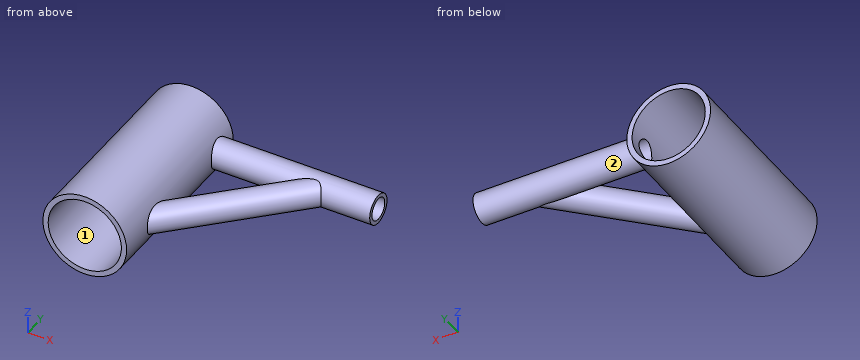
from build123d import *

# Parameters (mm, degrees)
F0_R          = 29.0718319872
F1_DEPTH      = 63.5
F3_D          = 50.8
F6_R          = 10.3012460199
F7_DEPTH      = 110.01212
F7_DEPTH_BACK = 2.28984
F11_START     = 10.10954
F10_R         = 9.3240211729
F11_DEPTH     = 116.89046
F13_D         = 15.24
F13_DEPTH     = 127
F13_TIP       = 4.578557917
F14_R         = 25.4
F15_DEPTH     = 127


with BuildPart() as f1:
    # F0 (on Front) → F1 (new body, symmetric)
    with BuildSketch(Plane.XZ):
        Circle(F0_R)
    extrude(amount=F1_DEPTH, both=True)

    # F3 (through all)
    with Locations(Plane.XZ.offset(63.5)):
        with Locations((0, 0)):
            Hole(F3_D / 2)

    # F6 (on plane+point) → F7 (join, two sides)
    with BuildSketch(Plane.YZ.offset(29.0718319872)) as f7_sk:
        with Locations((47.6702228189, 0)):
            Circle(F6_R)
    extrude(amount=F7_DEPTH)
    extrude(f7_sk.sketch, amount=-F7_DEPTH_BACK)

    # F10 (on line) → F11 (join)
    with BuildSketch(Plane(origin=(-16.7531975657, -16.7531975657, 0), x_dir=(-0.7071067812, 0.7071067812, 0), z_dir=(0.7071067812, 0.7071067812, 0)).offset(F11_START)):
        with Locations((-38.7535318732, 0)):
            Circle(F10_R)
    extrude(amount=F11_DEPTH)

    # F13
    with Locations(Plane.YZ.offset(139.0839519872)):
        with Locations((47.6702228189, 0)):
            Hole(F13_D / 2, depth=F13_DEPTH)
            with Locations((0, 0, -(F13_DEPTH + F13_TIP / 2))):  # 118° drill point
                Cone(0, F13_D / 2, F13_TIP, mode=Mode.SUBTRACT)

    # F14 (on Front) → F15 (cut)
    with BuildSketch(Plane.XZ):
        Circle(F14_R)
    extrude(amount=F15_DEPTH, mode=Mode.SUBTRACT)


solid = f1.part
Design review of the part built by this model. Coordinates are the model's own, in mm. Face numbers are marked on the shaded views. A direction names the side the tool comes from. Coordinates: 2 decimals unless noted, no trailing zeros. Loops run counter-clockwise (first coordinate to the right, second up) from the corner with the lowest first, then second, coordinate; pieces in that order, holes last. Notation, with made-up numbers: (8.25, 34.5) -> (64.25, 34.5) arc R11 ccw to (64.25, 38.5) -> close; hole circle Ø7 at (69.25, 1). An arc over 180 degrees is marked (long way). Use a Markdown table: item, result. Add a question column.
Item 1: We need section A-A, the plane z = -2.5. Write out the cut boundary in (x, y), and give its area (3 significant figures).
Item 2: We need section B-B, the plane x = 0. Write out the cut boundary in (y, z).
Item 3: We need section D-D, the plane y = -52. Write out the cut boundary in (x, z).
Item 4: We need section C-C, the plane z = 22. Write out the cut boundary in (x, y).
Item 5: Clearance check with flat-ended pins moving along their axes: P1, Ø12, axis at y = -30, z = -11.5, coming from the +X side; P2, Ø3, axis at x = 73, z = 4, coming from the +Y side; P3, Ø2, axis at x = 64, z = -6, coming from the -Y side. State where each tip first meets the part, or that it passes through.
Item 6: Wall thickness on L1, parallel to Y at x = 34.5, z = -3; L2, parallel to Z at x = 0, y = 3; L3, parallel to Y at x = 114, z = 0: over which ranges is each line inside the solid? List them lowest first. Write a range as from..to.
Item 7: Machinability: for the marked faces 1 and 2, which of the approach directions +Z, -Z, +X, -X, +Y, -Y give a long, thin tool a straight path to every point of the face, cutting with its end or side? Answer none if there is none.
Numbers:
| question | item | result |
|---|---|---|
| 1 | outline | (-28.96, -63.5) -> (-25.28, -63.5) -> (-25.28, 63.5) -> (-28.96, 63.5) -> close; (25.28, -63.5) -> (28.96, -63.5) -> (28.96, -38.54) -> (105.19, 37.68) -> (139.08, 37.68) -> (139.08, 40.47) -> (25.28, 40.47) -> close; (25.28, 54.87) -> (139.08, 54.87) -> (139.08, 57.66) -> (28.96, 57.66) -> (28.96, 63.5) -> (25.28, 63.5) -> close; hole (28.96, -13.14) -> (79.78, 37.68) -> (28.96, 37.68) -> close |
| 1 | area | 3,110 mm^2 |
| 2 | outline | (-63.5, -29.07) -> (63.5, -29.07) -> (63.5, -25.4) -> (-63.5, -25.4) -> close; (-63.5, 25.4) -> (63.5, 25.4) -> (63.5, 29.07) -> (-63.5, 29.07) -> close |
| 3 | outline | circle Ø58.14 at (0, 0); hole circle Ø50.8 at (0, 0) |
| 4 | outline | (-19, -63.5) -> (-12.69, -63.5) -> (-12.69, 63.5) -> (-19, 63.5) -> close; (12.69, -63.5) -> (19, -63.5) -> (19, 63.5) -> (12.69, 63.5) -> close |
| 5 | P1 | stops at x = 37.58 |
| 5 | P2 | stops at y = 57.66 |
| 5 | P3 | stops at y = -2.37 |
| 6 | L1 | y = -32.79..-7.82, 37.82..40.67, 54.67..57.52 |
| 6 | L2 | z = -29.07..-25.4, 25.4..29.07 |
| 6 | L3 | y = 37.37..40.05, 55.29..57.97 |
| 7 | face 1 | +Y, -Y |
| 7 | face 2 | none |
